The figure shows three views and two pictorial views of one solid part (mm, origin at its lowest corner). Answer the questions. Give positions to 0.01 mm unless a question says otherwise; leave off trailing zeros. Write each loop counter-clockwise with the first axis right and the second up, starting at its lowest first coordinate (ties: lowest second). Pieces come first, ordered by that corner, then holes. Notation, with made-up numbers: (85.5, 34) - (140.5, 34) arc R19 cw to (140.5, 44) - close; hole circle Ø1 at (81, 60.25). An arc over 180 degrees is marked (long way). One line per question, with ' | ' between items. Start each with the question number.
1. A cutting plane is placed at D-D (x = 47.5). Determine the outline of the cut face in (y, z), then the cut area to 3 significant figures.
2. The mould has two halves that part along X. Classify the marked faces 1, 2 and 3: +X half, -X half, draft (parallel to the pull), parting line (faces both ways), or undercut.
3. Given P1, Ø8, axis at x = 19.5, y = 21.5, coming from the +Z side, flat-ended and moving along its own axis, determine where the tip first touches the part or whether it passes through.
4. Find the intervals of material crossed by L1, parallel to Z at x = 32, y = 20.5 (1 decimal); L2, parallel to Z at x = 17, y = 10 (1 decimal); L3, parallel to Z at x = 8, y = 28.5, in increasing order. Write a range as from..to.
5. A cutting plane is placed at B-B (x = 32). Determine the outline of the cut face in (y, z), then the cut area to 3 significant figures.
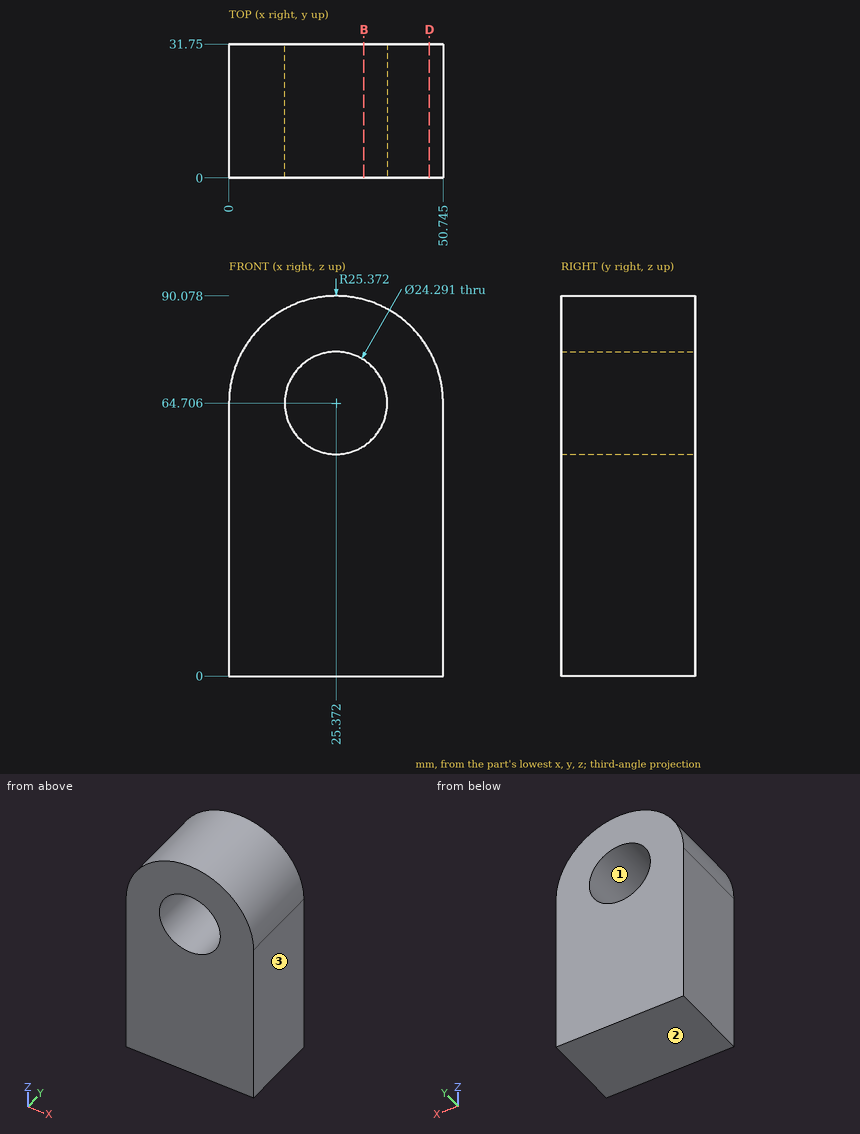
Determined:
1) outline: (0, 0) - (31.75, 0) - (31.75, 77.12) - (0, 77.12) - close | area: 2,450 mm2
2) face 1: undercut | face 2: draft | face 3: +X half
3) P1: z = 90.01
4) L1: 0..54.5, 74.9..89.2 | L2: 0..55.9, 73.5..88.7 | L3: 0..83.2
5) outline: (0, 0) - (31.75, 0) - (31.75, 54.53) - (0, 54.53) - close; (0, 74.88) - (31.75, 74.88) - (31.75, 89.2) - (0, 89.2) - close | area: 2,190 mm2
